```python
from build123d import *

# Parameters (mm, degrees)
F1_DEPTH  = 5.5
F3_DEPTH  = 3
F4_R      = 0.5
F5_DEPTH  = 1.125
F9_DEPTH  = 12.5
F10_W     = 14.8
F10_H     = 2.5
F11_DEPTH = 47
F13_DEPTH = 13.5
F14_R     = 0.5
F15_DEPTH = 4.25
F16_R     = 1
F17_DEPTH = 4.25


with BuildPart() as f1:
    # F0 (on Front) → F1 (new body)
    with BuildSketch(Plane.XZ):
        Polygon((0, -12.5), (0, 12.5), (-68.93, 12.5), (-68.93, -2.5), (-54, -2.5), (-54, -19.0381197846), (-54.8, -19.5), (-54.8, -47.5), (-48.1705947427, -44.1845815863), (-40, -12.5), align=None)
    extrude(amount=F1_DEPTH)

    # F2 (on face) → F3 (cut)
    with BuildSketch(Plane.XZ.offset(5.5)):
        Polygon((0, -8.25), (0, 8.25), (-54, 8.25), (-54, 31.9336503744), (-73.7788975239, 31.9336503744), (-73.7788975239, -2.5), (-54, -2.5), (-54, -8.25), align=None)
    extrude(amount=-F3_DEPTH, mode=Mode.SUBTRACT)

    # F4 (on face) → F5 (cut)
    with BuildSketch(Plane.XZ.offset(5.5)):
        with Locations((-4, 10.375)):
            Circle(F4_R)
        with Locations((-27, 10.375)):
            Circle(F4_R)
        with Locations((-50, 10.375)):
            Circle(F4_R)
        with Locations((-50, -10.375)):
            Circle(F4_R)
        with Locations((-27, -10.375)):
            Circle(F4_R)
        with Locations((-4, -10.375)):
            Circle(F4_R)
    extrude(amount=-F5_DEPTH, mode=Mode.SUBTRACT)

    # F8 (on offset) → F9 (cut)
    with BuildSketch(Plane.XY.offset(30)):
        Polygon((-67.1257596039, 0), (-62, -2.5), (-62, 0), align=None)
    extrude(amount=-F9_DEPTH, mode=Mode.SUBTRACT)

    # F10 (on face) → F11 (cut)
    with BuildSketch(Plane(origin=(0, 0, -12.5), x_dir=(1, 0, 0), z_dir=(0, 0, -1))):
        with Locations((-47.4, 1.25)):
            Rectangle(F10_W, F10_H)
    extrude(amount=F11_DEPTH, mode=Mode.SUBTRACT)

    # F12 (on plane+point) → F13 (cut)
    with BuildSketch(Plane(origin=(0, 0, -47.5), x_dir=(1, 0, 0), z_dir=(0, 0, -1))):
        Polygon((-48.6490884753, 5.5), (-54.8, 5.5), (-54.8, 2.5), align=None)
    extrude(amount=-F13_DEPTH, mode=Mode.SUBTRACT)

    # F14 (on face) → F15 (cut, through all)
    with BuildSketch(Plane.XY.offset(12.5)):
        with Locations((-7.54, -4)):
            Circle(F14_R)
        with Locations((-48.34, -4)):
            Circle(F14_R)
    extrude(amount=-F15_DEPTH, mode=Mode.SUBTRACT)

    # F16 (on face) → F17 (cut, through all)
    with BuildSketch(Plane.XY.offset(12.5)):
        with Locations((-27.94, -4)):
            Circle(F16_R)
    extrude(amount=-F17_DEPTH, mode=Mode.SUBTRACT)


solid = f1.part
```
The listing builds one solid part. Answer for the finished solid, in the listing's coordinates (mm). A direction names the side the tool comes from. Give positions to 0.01 mm unless a question says otherwise; leave off trailing zeros. Order: outer loops, then holes, each group sorted by start corner. A loop starts at its lowest first (then second) coordinate and runs counter-clockwise, first axis right, second up. Notation, with made-up numbers: (27, -13) -> (73, -13) arc R21 cw to (73, 22) -> close; hole circle Ø7 at (55.25, 28.5). An arc over 180 degrees is marked (long way). Answer as a JSON object with one key per item and string values. Group by question number.
Item 1: Flat-ended cylindrical pins translate along their axes: pin 1 (0.9 mm diameter, centred on x = -53, y = -4.5, fed in from -Z); pin 2 (0.5 mm diameter, centred on x = -4, z = -10.5, fed in from -Y) (3 decimals); pin 3 (0.8 mm diameter, centred on x = -4, z = 10, fed in from -Y); pin 4 (4.5 mm diameter, centred on x = -47.5, z = -29, fed in from +Y). Find the tip coordinate at first contact, or state that the pin passes through.
Item 2: The part is cut by section B-B on z = 2.5. Write down the section's boundary in (x, y), and give its area (3 significant figures).
Item 3: Determine the mould class of faces 4 (the flat face through (-44.14, -3.98, -28.56)), 5 (the flat face through (-27, -4, -8.25)), 6 (the flat face through (-51.77, -3.98, -39.34)) for opening direction Z: pulls with the +Z half, pulls with the -Z half, needs draft (parallel to the pull), parting line crosses it, or undercut.
Item 4: Consider L1, parallel to Y at x = -48.34, z = 11.1; L2, parallel to Z at x = -20, y = -3.4; L3, parallel to Z at x = -52, y = -4.3. Determine where each line is inside the solid, lowest interval first. Write a range as from..to.
Item 5: The part is cut by section C-C on x = -20.5. Write down the section's boundary in (y, z), and give its area (3 significant figures).
Item 6: The part is cut by section D-D on z = -5. Write down the section's boundary in (x, y), and give its area (3 significant figures).
Item 7: A tool of negligible diameter and unlimited length cuts with its end or side. For faces 1 (the flat face through (-62, -1, -2.5)), 2 (the flat face through (-49, -2.5, -26)), 3 (the flat face through (-54, -4, 10)), from which of +Z, -Z, +X, -X, +Y, -Y can it reach the whole face along a straight path? Write none if from no direction.
Item 8: The part is cut by section A-A on x = -42.5. Write down the section's boundary in (y, z), and give its area (3 significant figures).
Result set:
{
 "1": {"pin 1": "z = -34", "pin 2": "y = -4.375", "pin 3": "y = -5.5", "pin 4": "y = -2.5"},
 "2": {"outline": "(-68.93, -2.5) -> (0, -2.5) -> (0, 0) -> (-68.93, 0) -> close", "area": "172 mm²"},
 "3": {"face 4": "pulls with the -Z half", "face 5": "undercut", "face 6": "needs draft"},
 "4": {"L1": "-5.5..-4.5, -3.5..0", "L2": "-12.5..-8.25, 8.25..12.5", "L3": "-34..-8.25, 8.25..12.5"},
 "5": {"outline": "(-5.5, -12.5) -> (0, -12.5) -> (0, 12.5) -> (-5.5, 12.5) -> (-5.5, 8.25) -> (-2.5, 8.25) -> (-2.5, -8.25) -> (-5.5, -8.25) -> close", "area": "88.0 mm²"},
 "6": {"outline": "(-54, -2.5) -> (0, -2.5) -> (0, 0) -> (-54, 0) -> close", "area": "135 mm²"},
 "7": {"face 1": "-Z, -X, +Y, -Y", "face 2": "-Z, +X, -X, +Y", "face 3": "+Z, -X, -Y"},
 "8": {"outline": "(-5.5, -22.19) -> (-2.5, -22.19) -> (-2.5, -12.5) -> (0, -12.5) -> (0, 12.5) -> (-5.5, 12.5) -> (-5.5, 8.25) -> (-2.5, 8.25) -> (-2.5, -8.25) -> (-5.5, -8.25) -> close", "area": "117 mm²"}
}
